Part model, mm, in its own coordinate system. A direction names the side the tool comes from. Coordinates: 2 decimals unless noted, no trailing zeros. Write each loop counter-clockwise with the first axis right and the second up, starting at its lowest first coordinate (ties: lowest second). Pieces come first, ordered by that corner, then holes. Notation, with made-up numbers: (57.5, 9.25) -> (101.5, 9.25) arc R4 ccw to (101.5, 13.25) -> close; hole circle Ø6 at (61.25, 15). An arc over 180 degrees is marked (long way). One line per question, with ' | ' between items. Start each with the question number.
Item 1: Saw through at C-C (y = 2.5). List the corners of the cut face in (x, z) (1 decimal), and give its area (3 significant figures).
Item 2: Saw through at D-D (x = 47). List the corners of the cut face in (y, z) (3 decimals).
Item 3: Probe probe 1 along Z at (x, y) = (0, -4); probe 2 along Z at (x, y) = (28, -13.5); probe 3 along X at (y, z) = (-9, -6). List the from-to ranges inside material, lowest first. Write a range as [from, to].
Item 4: Pin check, flat tips, straight feed: pin 1 (5.5 mm diameter, centred on x = 5, z = 44.5, fed in from -Y); pin 2 (6 mm diameter, centred on y = -4.5, z = 33, fed in from +X); pin 3 (5 mm diameter, centred on x = -2, y = -10.5, fed in from +Z); pin 4 (17.5 mm diameter, centred on x = 33, y = -11.5, fed in from -Z). Stop position of each tip, or through.
Item 5: Saw through at B-B (z = 7). List the corners of the cut face in (x, y) (3 decimals), and give its area (3 significant figures).
Item 6: 3-axis set-ups, long thin cutter, end or side, ignore diameter. For faces 1 (the flat face through (-1, 0, -41)), 2 (the flat face through (-1, -8, 31.75)), 3 (the flat face through (16, 15.875, 1)): which of +Z, -Z, +X, -X, +Y, -Y reach the whole face in a straight line?
from build123d import *

# Parameters (mm, degrees)
F0_W     = 152.4
F0_H     = 63.5
F0_R     = 14.2875
F1_DEPTH = 15.875
F0_H_2   = 19.05
F2_DEPTH = 15.875


with BuildPart() as f1:
    # F0 (on Front) → F1 (new body)
    with BuildSketch(Plane.XZ):
        Rectangle(F0_W, F0_H)
        Circle(F0_R, mode=Mode.SUBTRACT)
    extrude(amount=F1_DEPTH)

    # F0 (on Front) → F2 (join)
    with BuildSketch(Plane.XZ):
        with Locations((0, 41.275)):
            Rectangle(F0_W, F0_H_2)
        Rectangle(F0_W, F0_H)
        Circle(F0_R, mode=Mode.SUBTRACT)
        with Locations((0, -41.275)):
            Rectangle(F0_W, F0_H_2)
    extrude(amount=-F2_DEPTH)


solid = f1.part
From the geometry:
1) outline: (-76.2, -50.8) -> (76.2, -50.8) -> (76.2, 50.8) -> (-76.2, 50.8) -> close; hole circle Ø28.6 at (0, 0) | area: 14,800 mm2
2) outline: (-15.875, -31.75) -> (0, -31.75) -> (0, -50.8) -> (15.875, -50.8) -> (15.875, 50.8) -> (0, 50.8) -> (0, 31.75) -> (-15.875, 31.75) -> close
3) probe 1: [-31.75, -14.29], [14.29, 31.75] | probe 2: [-31.75, 31.75] | probe 3: [-76.2, -12.97], [12.97, 76.2]
4) pin 1: y = 0 | pin 2: x = 76.2 | pin 3: z = 31.75 | pin 4: z = -31.75
5) outline: (-76.2, -15.875) -> (-12.455, -15.875) -> (-12.455, 15.875) -> (-76.2, 15.875) -> close; (12.455, -15.875) -> (76.2, -15.875) -> (76.2, 15.875) -> (12.455, 15.875) -> close | area: 4,050 mm2
6) face 1: -Z, +X, -X, -Y | face 2: +Z, +X, -X, -Y | face 3: +Z, -Z, +X, -X, +Y
